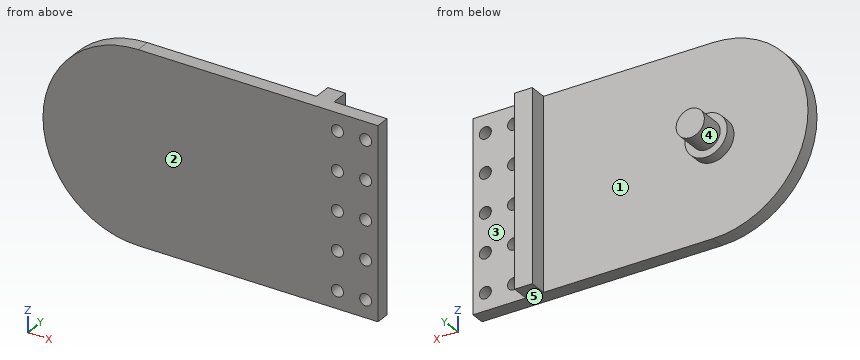
Autodesk Inventor part; units mm, degrees
ref_plane "YZ Plane" through (0, 0, 0) normal (1, 0, 0) x (0, 1, 0)
ref_plane "XZ Plane" through (0, 0, 0) normal (0, 1, 0) x (-1, 0, 0)
ref_plane "XY Plane" through (0, 0, 0) normal (0, 0, 1) x (1, 0, 0)
sketch "Skizze1" plane through (0, 0, 0) normal (0, 1, 0) x (-1, 0, 0)
  line L0 (-50, 27) -> (50, 27)
  line L1 (50, 27) -> (50, -27) construction
  line L2 (50, -27) -> (-50, -27)
  line L3 (-50, -27) -> (-50, 27)
  line L4 (-50, 27) -> (50, -27) construction
  line L5 (50, 27) -> (-50, -27) construction
  line L6 (0, 0) -> (66.4326, 0) construction
  arc A0 (18, -27) -> (18, 27) centre (18, 0) ccw
  dimension "d0" = 54
  dimension "d1" = 100
  dimension "d12" = 68
  dimension "d13" = 90
extrude "Extrusion1" add sketch "Skizze1" along normal blind 4
sketch "Skizze3" plane through (0, 4, 0) normal (0, 1, 0) x (1, 0, 0)
  circle A0 centre (-18, 0) radius 6
  line L0 (0, 0) -> (-17.1865, 0) construction
  line L1 (50, -27) -> (50, 27) construction
  line L2 (-18, -27) -> (50, -27)
  line L3 (50, -27) -> (50, 27) construction
  line L4 (50, 27) -> (-18, 27) construction
  line L5 (-18, -27) -> (50, -27) construction
  line L6 (50, 27) -> (-18, 27) construction
  arc A1 (-18, 27) -> (-18, -27) centre (-18, 0) ccw
  point P0 (-50, -27)
  point P1 (-50, 27)
  dimension "d8" = 12
  dimension "d9" = 68
extrude "Extrusion3" [suppressed]
sketch "Skizze5" plane through (0, 4, 0) normal (0, 1, 0) x (1, 0, 0)
  line L0 (-18, -27) -> (50, -27)
  line L1 (50, -27) -> (50, 27)
  line L2 (50, 27) -> (-18, 27)
  arc A0 (-18, 27) -> (-18, -27) centre (-18, 0) ccw
  line L3 (35, -27) -> (30, -27)
  line L4 (30, -27) -> (30, 27)
  line L5 (30, 27) -> (35, 27)
  line L6 (35, 27) -> (35, -27)
  point P0 (0, 0)
  dimension "d14" = 15
  dimension "d15" = 5
extrude "Extrusion4" add sketch "Skizze5" along normal blind 5 contours L4 L2 L6 L0
sketch "Skizze6" plane through (0, 4, 0) normal (0, 1, 0) x (1, 0, 0)
  line L0 (35, 27) -> (35, -27)
  line L1 (35, -27) -> (50, -27)
  line L2 (50, -27) -> (50, 27)
  line L3 (50, 27) -> (35, 27)
  line L4 (0, 0) -> (67.4565, 0) construction
  point P0 (46.5, 0)
  dimension "d18" = 3.5
hole "Bohrung1" at (46.5, 4, 0) direction (0, -1, 0) diameter 3.4 end through all
pattern_linear "Rechteckige Anordnung1" count 5 spacing 11 along (0, 0, -1) count 2 spacing 8 along (-1, 0, 0) of "Bohrung1" first direction both ways yes
sketch "Skizze7" plane through (0, 0, 0) normal (0, -1, 0) x (1, 0, 0)
  circle A0 centre (-18, 0) radius 6
  circle A1 centre (-18, 0) radius 10 construction
  line L0 (-18, -12.7159) -> (-18, 15.8855)
  line L1 (-33.0539, 0) -> (-6.7164, 0)
  point P0 (0, 0)
  point P1 (-18, -10)
  point P2 (-28, 0)
  point P3 (-18, 10)
  point P4 (-8, 0)
  dimension "d32" = 20
hole "Bohrung2" [suppressed]
sketch "Skizze8" plane through (0, 4, 0) normal (0, 1, 0) x (1, 0, 0)
  arc A0 (-18, 27) -> (-18, -27) centre (-18, 0) ccw
  circle A1 centre (-18, 0) radius 6
  circle A2 centre (-18, 0) radius 4
  point P0 (0, 0)
  dimension "d40" = 12
  dimension "d43" = 8
extrude "Extrusion5" add sketch "Skizze8" along normal blind 3 contours A1 | A2
extrude "Extrusion6" add sketch "Skizze8" along normal blind 10 contours A2
properties part number "dynamixel_pro_frame_part2" material "Aluminium 6061"
Model file for the job. Use its own axes, mm. Face numbers are marked on the shaded views. A direction names the side the tool comes from. Give positions to 0.01 mm unless a question says otherwise; leave off trailing zeros. Loops run counter-clockwise (first coordinate to the right, second up) from the corner with the lowest first, then second, coordinate; pieces in that order, holes last. Notation, with made-up numbers: M 82.25,43 L 139.25,43 A15 cw 139.25,56 Z; hole C 27.5,58 d7. An arc over 180 degrees is marked long. Use one line per item in the form item = value.
Item 1: Drill centre lines: L1, parallel to Z at x = 46.5, y = 2.25; L2, parallel to X at y = 2.05, z = 0; L3, parallel to X at y = 1.1, z = 11. Where is each one in solid material? Low to high.
Filled in:
L1 = -27 to -23.7, -20.3 to -12.7, -9.3 to -1.7, 1.7 to 9.3, 12.7 to 20.3, 23.7 to 27
L2 = -45 to 36.8, 40.2 to 44.8, 48.2 to 50
L3 = -42.66 to 36.8, 40.2 to 44.8, 48.2 to 50
Item 2: Slice it at B-B on y = 3. Give the number of separate pieces and of enclosed holes in the cut face, and give its area (3 significant figures).
Filled in:
separate_pieces = 1
enclosed_holes = 10
area = 4,730 mm^2
Item 3: Slice it at A-A on z = 0. List the corners of the cut face in (x, y).
Filled in:
outline = M -45,0 L 36.8,0 L 36.8,4 L 35,4 L 35,9 L 30,9 L 30,4 L -12,4 L -12,7 L -14,7 L -14,14 L -22,14 L -22,7 L -24,7 L -24,4 L -45,4 Z; M 40.2,0 L 44.8,0 L 44.8,4 L 40.2,4 Z; M 48.2,0 L 50,0 L 50,4 L 48.2,4 Z
Item 4: Slice it at C-C on x = 38.5. List the corners of the cut face in (y, z), and give its area (3 significant figures).
Filled in:
outline = M 0,-27 L 4,-27 L 4,-23.7 L 0,-23.7 Z; M 0,-20.3 L 4,-20.3 L 4,-12.7 L 0,-12.7 Z; M 0,-9.3 L 4,-9.3 L 4,-1.7 L 0,-1.7 Z; M 0,1.7 L 4,1.7 L 4,9.3 L 0,9.3 Z; M 0,12.7 L 4,12.7 L 4,20.3 L 0,20.3 Z; M 0,23.7 L 4,23.7 L 4,27 L 0,27 Z
area = 148 mm^2
Item 5: Flat gauge pins, fed straight in: pin 1 Ø12 at (x, z) = (40.5, -2) entering from +Y; pin 2 Ø5.5 at (x, z) = (38.5, 22) entering from +Y; pin 3 Ø5.5 at (y, z) = (6, 11.5) entering from -X. Where does each tip first touch, or does it go through?
Filled in:
pin_1 = 9
pin_2 = 4
pin_3 = -43.23
Item 6: Which spindle directions (+Z, -Z, +X, -X, +Y, -Y) get a long thin tool onto all of the face, cutting with end or side? Do the marked faces 3, 4 and 5. Say none if no direction does.
Filled in:
face_3 = +Z, -Z, +X, +Y
face_4 = +Y
face_5 = -Z, +X, -X, +Y, -Y
Item 7: Two-plate mould, pull along X, no slides. Class the marked faces 1 and 2: released by +X, released by -X, zero draft, split by the parting line, or undercut.
Filled in:
face_1 = undercut
face_2 = zero draft
Item 8: Slice it at D-D on x = -19.5. List the corners of the cut face in (y, z), and give its area (3 significant figures).
Filled in:
outline = M 0,-26.96 L 4,-26.96 L 4,-5.81 L 7,-5.81 L 7,-3.71 L 14,-3.71 L 14,3.71 L 7,3.71 L 7,5.81 L 4,5.81 L 4,26.96 L 0,26.96 Z
area = 302 mm^2
